CAD build for the part. Positions are in the model's coordinates, mm. A direction names the side the tool comes from. Give positions to 0.01 mm unless a question says otherwise; leave off trailing zeros. Loops run counter-clockwise (first coordinate to the right, second up) from the corner with the lowest first, then second, coordinate; pieces in that order, holes last. Notation, with made-up numbers: M 77.25,0.5 L 125.25,0.5 A22 cw 125.25,29.5 Z; hole C 85.25,63.25 d1. An arc over 180 degrees is marked long. Answer as CSV lines item,"result".
```python
from build123d import *

# Parameters (mm, degrees)
BOSS_EXTRUDE1_DEPTH            = 7
BOSS_EXTRUDE2_DEPTH            = 25
SKETCH2_R                      = 2.275
CUT_EXTRUDE1_DEPTH             = 6
CBORE_FOR_M3_SHCS1_D           = 3.4
CBORE_FOR_M3_SHCS1_DEPTH       = 7
CBORE_FOR_M3_SHCS1_CBORE_D     = 6.5
CBORE_FOR_M3_SHCS1_CBORE_DEPTH = 3
CBORE_FOR_M3_SHCS1_TIP         = 1.021463052
CUT_EXTRUDE2_DEPTH             = 125.119013182
CUT_EXTRUDE2_DEPTH_BACK        = 125.119013182
SKETCH5_W                      = 69.118587288
SKETCH5_H                      = 18
SKETCH6_W                      = 2.4
SKETCH6_H                      = 56.748995089
CUT_EXTRUDE3_DEPTH             = 95.024950421
SKETCH7_R                      = 2.275
BOSS_EXTRUDE3_DEPTH            = 3
CHAMFER1_SIZE                  = 0.5


with BuildPart() as part:
    # Sketch1 → Boss-Extrude1 (new body)
    with BuildSketch(Plane(origin=(0, 0, -11.1516868), x_dir=(-1, 0, 0), z_dir=(0, 0, -1))):
        with BuildLine():
            Line((-25.216678302, 125.2267128), (-25.216678302, 68.477717711))
            ThreePointArc((-25.216678302, 68.477717711), (-25.796051859, 67.07898621), (-27.19478336, 66.499612653))
            Line((-27.19478336, 66.499612653), (-113.777448917, 66.499612653))
            ThreePointArc((-113.777448917, 66.499612653), (-115.166333777, 67.074907598), (-115.741628722, 68.463792459))
            Line((-115.741628722, 68.463792459), (-115.741628722, 125.322842242))
            ThreePointArc((-115.741628722, 125.322842242), (-115.174757862, 126.691389562), (-113.806210541, 127.258260423))
            Line((-113.806210541, 127.258260423), (-27.248225925, 127.258260423))
            ThreePointArc((-27.248225925, 127.258260423), (-25.811704824, 126.6632339), (-25.216678302, 125.2267128))
        make_face()
    extrude(amount=-BOSS_EXTRUDE1_DEPTH)

    # Sketch1<4> → Boss-Extrude2 (add)
    with BuildSketch(Plane(origin=(0, 0, -11.1516868), x_dir=(-1, 0, 0), z_dir=(0, 0, -1))):
        with BuildLine():
            Line((-22.216678302, 125.2267128), (-22.216678302, 68.477717711))
            ThreePointArc((-22.216678302, 68.477717711), (-23.674731516, 64.957665867), (-27.19478336, 63.499612653))
            Line((-27.19478336, 63.499612653), (-113.777448917, 63.499612653))
            ThreePointArc((-113.777448917, 63.499612653), (-117.28765412, 64.953587255), (-118.741628722, 68.463792459))
            Line((-118.741628722, 68.463792459), (-118.741628722, 125.322842242))
            ThreePointArc((-118.741628722, 125.322842242), (-117.296078205, 128.812709906), (-113.806210541, 130.258260423))
            Line((-113.806210541, 130.258260423), (-27.248225925, 130.258260423))
            ThreePointArc((-27.248225925, 130.258260423), (-23.690384481, 128.784554244), (-22.216678302, 125.2267128))
        make_face()
        with BuildLine():
            Line((-25.216678302, 125.2267128), (-25.216678302, 68.477717711))
            ThreePointArc((-25.216678302, 68.477717711), (-25.796051859, 67.07898621), (-27.19478336, 66.499612653))
            Line((-27.19478336, 66.499612653), (-113.777448917, 66.499612653))
            ThreePointArc((-113.777448917, 66.499612653), (-115.166333777, 67.074907598), (-115.741628722, 68.463792459))
            Line((-115.741628722, 68.463792459), (-115.741628722, 125.322842242))
            ThreePointArc((-115.741628722, 125.322842242), (-115.174757862, 126.691389562), (-113.806210541, 127.258260423))
            Line((-113.806210541, 127.258260423), (-27.248225925, 127.258260423))
            ThreePointArc((-27.248225925, 127.258260423), (-25.811704824, 126.6632339), (-25.216678302, 125.2267128))
        make_face(mode=Mode.SUBTRACT)
    extrude(amount=-BOSS_EXTRUDE2_DEPTH)

    # Sketch2 → Cut-Extrude1 (cut)
    with BuildSketch(Plane.XY.offset(-4.1516868)):
        with Locations((111.633, 123.952)):
            Circle(SKETCH2_R)
        with Locations((111.633, 69.901)):
            Circle(SKETCH2_R)
        with Locations((29.083, 69.901)):
            Circle(SKETCH2_R)
        with Locations((29.083, 123.952)):
            Circle(SKETCH2_R)
    extrude(amount=-CUT_EXTRUDE1_DEPTH, mode=Mode.SUBTRACT)

    # CBORE for M3 SHCS1
    with Locations(Plane.XY.offset(-4.1516868)):
        with Locations((55.506677482, 96.899230975), (85.506670618, 96.878936538)):
            CounterBoreHole(CBORE_FOR_M3_SHCS1_D / 2, CBORE_FOR_M3_SHCS1_CBORE_D / 2, CBORE_FOR_M3_SHCS1_CBORE_DEPTH, depth=CBORE_FOR_M3_SHCS1_DEPTH)
            with Locations((0, 0, -(CBORE_FOR_M3_SHCS1_DEPTH + CBORE_FOR_M3_SHCS1_TIP / 2))):  # 118° drill point
                Cone(0, CBORE_FOR_M3_SHCS1_D / 2, CBORE_FOR_M3_SHCS1_TIP, mode=Mode.SUBTRACT)

    # Sketch5 → Cut-Extrude2 (cut, two sides: drawn at the far end of the back side and taken through both)
    with BuildSketch(Plane(origin=(0, 96.878936538, 0), x_dir=(-1, 0, 0), z_dir=(0, -1, 0)).offset(-CUT_EXTRUDE2_DEPTH_BACK)):
        with Locations((-62.563646937, -4.8483132)):
            Rectangle(SKETCH5_W, SKETCH5_H)
    extrude(amount=CUT_EXTRUDE2_DEPTH + CUT_EXTRUDE2_DEPTH_BACK, mode=Mode.SUBTRACT)

    # Sketch6 → Cut-Extrude3 (cut)
    with BuildSketch(Plane(origin=(22.216678302, -0.007433612, 0), x_dir=(0, 0, 1), z_dir=(-1, 0, 0))):
        with Locations((11.1483132, 96.859648867)):
            Rectangle(SKETCH6_W, SKETCH6_H)
        Polygon((12.3483132, 127.265694035), (11.1483132, 128.765694035), (9.9483132, 127.265694035), (9.9483132, 125.234146412), (12.3483132, 125.234146412), align=None)
        Polygon((12.3483132, 68.485151323), (9.9483132, 68.485151323), (9.9483132, 66.507046265), (11.1483132, 64.953603699), (12.3483132, 66.507046265), align=None)
    extrude(amount=-CUT_EXTRUDE3_DEPTH, mode=Mode.SUBTRACT)

    # Sketch7 → Boss-Extrude3 (add)
    # profile 1 of 4: a face of its own
    with BuildSketch(Plane.XY.offset(-4.1516868)):
        with BuildLine():
            Line((25.216678302, 125.2267128), (25.216678302, 118.952))
            Line((25.216678302, 118.952), (34.083, 118.952))
            Line((34.083, 118.952), (34.083, 130.258260423))
            Line((34.083, 130.258260423), (28.004353293, 130.258260423))
            Line((28.004353293, 130.258260423), (28.004353293, 127.258260423))
            Line((28.004353293, 127.258260423), (27.248225925, 127.258260423))
            ThreePointArc((27.248225925, 127.258260423), (25.811704824, 126.6632339), (25.216678302, 125.2267128))
        make_face()
        with Locations((29.083, 123.952)):
            Circle(SKETCH7_R, mode=Mode.SUBTRACT)
    # profile 2 of 4: a face of its own
    with BuildSketch(Plane.XY.offset(-4.1516868)):
        with BuildLine():
            Line((34.083, 74.901), (25.216678302, 74.901))
            Line((25.216678302, 74.901), (25.216678302, 68.477717711))
            ThreePointArc((25.216678302, 68.477717711), (25.796051859, 67.07898621), (27.19478336, 66.499612653))
            Line((27.19478336, 66.499612653), (28.004353293, 66.499612653))
            Line((28.004353293, 66.499612653), (28.004353293, 63.499612653))
            Line((28.004353293, 63.499612653), (34.083, 63.499612653))
            Line((34.083, 63.499612653), (34.083, 74.901))
        make_face()
        with Locations((29.083, 69.901)):
            Circle(SKETCH7_R, mode=Mode.SUBTRACT)
    # profile 3 of 4: a face of its own
    with BuildSketch(Plane.XY.offset(-4.1516868)):
        with BuildLine():
            Line((106.633, 118.952), (115.741628722, 118.952))
            Line((115.741628722, 118.952), (115.741628722, 125.322842242))
            ThreePointArc((115.741628722, 125.322842242), (115.174757862, 126.691389562), (113.806210541, 127.258260423))
            Line((113.806210541, 127.258260423), (106.633, 127.258260423))
            Line((106.633, 127.258260423), (106.633, 118.952))
        make_face()
        with Locations((111.633, 123.952)):
            Circle(SKETCH7_R, mode=Mode.SUBTRACT)
    # profile 4 of 4: a face of its own
    with BuildSketch(Plane.XY.offset(-4.1516868)):
        with BuildLine():
            Line((115.741628722, 68.463792459), (115.741628722, 74.901))
            Line((115.741628722, 74.901), (106.633, 74.901))
            Line((106.633, 74.901), (106.633, 66.499612653))
            Line((106.633, 66.499612653), (113.777448917, 66.499612653))
            ThreePointArc((113.777448917, 66.499612653), (115.166333777, 67.074907598), (115.741628722, 68.463792459))
        make_face()
        with Locations((111.633, 69.901)):
            Circle(SKETCH7_R, mode=Mode.SUBTRACT)
    extrude(amount=BOSS_EXTRUDE3_DEPTH)

    # Chamfer1
    chamfer1_edges = [part.edges().sort_by_distance(p)[0] for p in [
        (26.808, 69.901, -1.1516868),
        (109.358, 123.952, -1.1516868),
        (109.358, 69.901, -1.1516868),
        (26.808, 123.952, -1.1516868),
    ]]
    chamfer(chamfer1_edges, length=CHAMFER1_SIZE)


solid = part.part
```
Q1. Which spindle directions (+Z, -Z, +X, -X, +Y, -Y) get a long thin tool onto all of the face, cutting with end or side? Do faces 4 (the cylindrical face through (85.88, 95.22, -9.18)), 5 (the flat face through (24, 96, 12.348)), 6 (the cylindrical face through (82.93, 94.9, -5.63)), 7 (the flat face through (28.004, 129, 6)). Say none if no direction does.
Solution:
face 4,"+Z, -Z"
face 5,"-X"
face 6,"+Z"
face 7,"+Z, +Y, -Y"
Q2. Mould opens along X. For faces 1 (the flat face through (28.004, 65, 6)), 2 (the cylindrical face through (23.636, 64.997, 1.173)), 3 (the flat face through (116, 97, 9.948)) say: released by +X, released by -X, zero draft, split by the parting line, or undercut.
Solution:
face 1,"undercut"
face 2,"released by -X"
face 3,"zero draft"
Q3. Cut at A-A (y = 115.5). Write the cut outline in (x, z).
Solution:
outline,"M 22.22,-11.15 L 118.74,-11.15 L 118.74,13.85 L 115.74,13.85 L 115.74,12.35 L 117.24,12.35 L 117.24,9.95 L 115.74,9.95 L 115.74,-4.15 L 25.22,-4.15 L 25.22,9.95 L 22.22,9.95 Z; M 22.22,12.35 L 25.22,12.35 L 25.22,13.85 L 22.22,13.85 Z"
Q4. Cut at B-B (z = 1.5). Write the cut outline in (x, y), and give its area (3 significant figures).
Solution:
outline,"M 22.22,68.48 A4.98 ccw 27.19,63.5 L 28,63.5 L 28,66.5 L 27.19,66.5 A1.98 cw 25.22,68.48 L 25.22,125.23 A2.03 cw 27.25,127.26 L 28,127.26 L 28,130.26 L 27.25,130.26 A5.03 ccw 22.22,125.23 Z; M 97.12,63.5 L 113.78,63.5 A4.96 ccw 118.74,68.46 L 118.74,125.32 A4.94 ccw 113.81,130.26 L 97.12,130.26 L 97.12,127.26 L 113.81,127.26 A1.94 cw 115.74,125.32 L 115.74,68.46 A1.96 cw 113.78,66.5 L 97.12,66.5 Z"
area,"511 mm²"
Q5. Wall check: line 1 (X direction, y = 104, z = 2.75); line 2 (X direction, y = 125.5, z = -9.25); line 3 (X direction, y = 70.5, z = -7.25). Give the ranges that are in metal, low to high. Write a range as [from, to].
Solution:
line 1,"x = [22.22, 25.22], [115.74, 118.74]"
line 2,"x = [22.22, 27.42], [30.75, 109.97], [113.3, 118.74]"
line 3,"x = [22.22, 26.89], [31.28, 109.44], [113.83, 118.74]"
Q6. Pin check, flat tips, straight feed: P1, Ø12, axis at x = 104, y = 82, coming from the +Z side; P2, Ø5, axis at x = 106.5, y = 121.5, coming from the +Z side; P3, Ø3, axis at x = 86.5, y = 98, coming from the +Z side. Stop position of each tip, or through.
Solution:
P1,"stops at z = -4.15"
P2,"stops at z = -1.15"
P3,"stops at z = -7.15"
Q7. Cut at C-C (x = 38). Write the cut outline in (y, z), and give its area (3 significant figures).
Solution:
outline,"M 63.5,-11.15 L 130.26,-11.15 L 130.26,-4.15 L 63.5,-4.15 Z"
area,"467 mm²"
